Autodesk Inventor part; units mm, degrees
ref_plane "YZ Plane" through (0, 0, 0) normal (1, 0, 0) x (0, 1, 0)
ref_plane "XZ Plane" through (0, 0, 0) normal (0, 1, 0) x (-1, 0, 0)
ref_plane "XY Plane" through (0, 0, 0) normal (0, 0, 1) x (1, 0, 0)
sketch "Szkic1" plane through (0, 0, 0) normal (0, 1, 0) x (-1, 0, 0)
  line L0 (1.25, 50) -> (-1.25, 50)
  line L1 (-11.25, 40) -> (-11.25, -40)
  line L2 (-1.25, -50) -> (1.25, -50)
  line L3 (11.25, -40) -> (11.25, 40)
  line L4 (11.25, 50) -> (-11.25, -50)
  line L5 (11.25, -50) -> (-11.25, 50)
  arc A0 (11.25, 40) -> (1.25, 50) centre (1.25, 40) ccw
  arc A1 (-1.25, 50) -> (-11.25, 40) centre (-1.25, 40) ccw
  arc A2 (1.25, -50) -> (11.25, -40) centre (1.25, -40) ccw
  arc A3 (-11.25, -40) -> (-1.25, -50) centre (-1.25, -40) ccw
  point P0 (0, 0)
  point P1 (0, 0)
  dimension "d0" = 22.5
  dimension "d1" = 100
  dimension "d2" = 10
extrude "Wyciągnięcie proste1" add sketch "Szkic1" along normal blind 4.1
sketch "Szkic2" plane through (0, 4.1, 0) normal (0, 1, 0) x (1, 0, 0)
  circle A0 centre (0, 44) radius 3.5
  line L0 (1.25, 50) -> (-1.25, 50)
  point P0 (0, 0)
  point P1 (0, 50)
  dimension "d5" = 7
  dimension "d14" = 6
extrude "Wyciągnięcie proste2" cut sketch "Szkic2" against normal blind 8
sketch "Szkic3" plane through (0, 4.1, 0) normal (0, 1, 0) x (1, 0, 0)
  line L0 (0, 47.5) -> (0, 28.5)
  arc A0 (-2, 28.5) -> (2, 28.5) centre (0, 28.5) ccw
  line L1 (-2.75, 41.8349) -> (0, 41.8349)
  line L2 (1.25, 50) -> (-1.25, 50)
  line L3 (-2, 28.5) -> (-2.75, 41.8349)
  line L4 (2, 28.5) -> (2.75, 41.8349)
  line L5 (0, 41.8349) -> (2.75, 41.8349)
  circle A1 centre (0, 44) radius 3.5
  point P0 (0, 0)
  point P1 (0, 50)
  dimension "d8" = 19
  dimension "d10" = 5.5
  dimension "d22" = 13.3349
extrude "Wyciągnięcie proste3" cut sketch "Szkic3" against normal blind 1.1 contours L5 A1 L0 | L0 A1 L1 | A1 L4 A0 L3 picked at (1.6483, 41.6479) picked at (-1.6483, 41.6479)
sketch "Szkic9" plane through (0, 4.1, 0) normal (0, 1, 0) x (1, 0, 0)
  line L0 (-1.25, -50) -> (1.25, -50)
  line L1 (11.25, -40) -> (11.25, -23)
  line L2 (11.25, -23) -> (-11.25, -23)
  line L3 (-11.25, -23) -> (-11.25, -40)
  line L4 (-1.25, -50) -> (1.25, -50)
  arc A0 (-11.25, -40) -> (-1.25, -50) centre (-1.25, -40) ccw
  arc A1 (1.25, -50) -> (11.25, -40) centre (1.25, -40) ccw
  point P0 (0, 0)
  point P1 (0, -50)
  dimension "d36" = 27
  dimension "d37" = 22.5
  dimension "d38" = 10
extrude "Wyciągnięcie proste7" add sketch "Szkic9" along normal blind 3.7
properties part number "arm_big_part_v2"
Check sheet for the modelled part. Datum: model origin and axes. Units: mm. A direction names the side the tool comes from. Round coordinates to 2 decimals unless told otherwise and drop trailing zeros. Order: outer loops, then holes, each group sorted by start corner. A loop starts at its lowest first (then second) coordinate and runs counter-clockwise, first axis right, second up. Notation, with made-up numbers: M 15,6.5 L 58,6.5 A16 cw 58,33.5 Z; hole C -19,8 d6. An arc over 180 degrees is marked long. Answer in a Markdown table with one row per item.
(1) Draft check along X on faces 1 (the cylindrical face through (-0.46, 2.08, -47.47)), 2 (the flat face through (-11.25, 3, 8)), 3 (the cylindrical face through (0, 3.6, -26.5)), 4 (the flat face through (0, 6, 23)). Enter one of: +X half, -X half, draft (parallel to the pull), parting line (faces both ways), or undercut.
Findings:
| item | result |
|---|---|
| face 1 | undercut |
| face 2 | -X half |
| face 3 | undercut |
| face 4 | draft |
(2) Section check C-C on y = 6. Record the boundary of the cut face in (x, z), plus the area to 3 significant figures.
Findings:
| item | result |
|---|---|
| outline | M -11.25,23 L 11.25,23 L 11.25,40 A10 ccw 1.25,50 L -1.25,50 A10 ccw -11.25,40 Z |
| area | 565 mm^2 |
(3) Material ranges on line 1 along Z through (x, y) = (0, 3.15); line 2 along X through (y, z) = (3.25, -28.5); line 3 along Z through (x, y) = (0, 2.15), recorded low to high. Write a range as from..to.
Findings:
| item | result |
|---|---|
| line 1 | z = -50..-47.5, -26.5..50 |
| line 2 | x = -11.25..-2, 2..11.25 |
| line 3 | z = -50..-47.5, -40.5..50 |
(4) Section check D-D on z = -44. Record the boundary of the cut face in (x, y), plus the area to 3 significant figures.
Findings:
| item | result |
|---|---|
| outline | M -10.42,0 L -3.5,0 L -3.5,4.1 L -10.42,4.1 Z; M 3.5,0 L 10.42,0 L 10.42,4.1 L 3.5,4.1 Z |
| area | 56.7 mm^2 |
(5) Gauge pin test, flat ends, axial feed: pin 1 (3 mm diameter, centred on x = 0, z = -30.5, fed in from +Y); pin 2 (5.5 mm diameter, centred on x = 0, z = -44, fed in from +Y); pin 3 (1.1 mm diameter, centred on x = -0.5, y = 6, fed in from -Z); pin 4 (11 mm diameter, centred on x = 4, z = -31.5, fed in from +Y). Record the tip position at first contact, or that the pin passes through.
Findings:
| item | result |
|---|---|
| pin 1 | stops at y = 3 |
| pin 2 | passes through |
| pin 3 | stops at z = 23 |
| pin 4 | stops at y = 4.1 |
(6) Section check A-A on x = 0. Record the boundary of the cut face in (y, z), plus the area to 3 significant figures.
Findings:
| item | result |
|---|---|
| outline | M 0,-50 L 4.1,-50 L 4.1,-47.5 L 0,-47.5 Z; M 0,-40.5 L 3,-40.5 L 3,-26.5 L 4.1,-26.5 L 4.1,23 L 7.8,23 L 7.8,50 L 0,50 Z |
| area | 466 mm^2 |
(7) Section check B-B on y = 1.25. Record the boundary of the cut face in (x, z), plus the area to 3 significant figures.
Findings:
| item | result |
|---|---|
| outline | M -11.25,-40 A10 ccw -1.25,-50 L 1.25,-50 A10 ccw 11.25,-40 L 11.25,40 A10 ccw 1.25,50 L -1.25,50 A10 ccw -11.25,40 Z; hole C 0,-44 d7 |
| area | 2,130 mm^2 |
(8) Set-up check for faces 5 (the cylindrical face through (-8.4, 2.02, -46.99)), 6 (the flat face through (0, 3, -34)), 7 (the flat face through (0, 4.1, -13)): record each of +Z, -Z, +X, -X, +Y, -Y from which the full face is reachable in a straight line by a thin tool's end or side.
Findings:
| item | result |
|---|---|
| face 5 | -Z, -X, +Y, -Y |
| face 6 | +Y |
| face 7 | -Z, +X, -X, +Y |
